Autodesk Fusion 360 part; units mm, degrees
sketch "Sketch1" plane through (0, 0, 0) normal (0, 0, 1) x (1, 0, 0)
  line L0 (0.0319, -0.0588) -> (7.7319, -0.0588)
  line L1 (0.0319, 17.6912) -> (0.0319, -0.0588)
  line L2 (0.0319, 17.6912) -> (5.3319, 17.6912)
  line L3 (0.0319, 8.7412) -> (4.5319, 8.7412)
  line L4 (4.5319, 10.9412) -> (0.0319, 10.9412)
  spline S0 degree 5 poles (5.3319, 17.6912) (5.3878, 17.5532) (5.4935, 17.2775) (5.633, 16.8647) (5.7805, 16.3159) (5.8962, 15.6328) (5.9374, 14.9527) (5.8981, 14.2761) (5.7753, 13.6028) (5.5729, 12.9329) (5.297, 12.2661) (5.0223, 11.7348) (4.7879, 11.3376) (4.6193, 11.0732) (4.5319, 10.9412) knots 0 0 0 0 0 0 0.1 0.2 0.3 0.4 0.5 0.6 0.7 0.8 0.9 1 1 1 1 1 1
  line L5 (0.0319, 10.9412) -> (4.5319, 10.9412)
  arc A0 (7.7319, -0.0588) -> (4.5319, 8.7412) centre (-3.0926, 0.9869) ccw
  line L6 (4.5319, 8.7412) -> (4.5319, 10.9412)
  line L7 (0.0319, 10.9412) -> (0.0319, 8.7412)
  line L8 (0.0319, 10.9412) -> (0.0319, 8.7412)
  line L9 (0.0319, 14.3162) -> (5.8819, 14.3162)
  line L10 (0.0319, 17.6912) -> (0.0319, 10.9412)
  line L11 (7.7319, -0.0588) -> (7.9819, -0.0588)
  line L12 (4.5319, 8.7412) -> (4.7819, 8.7412)
  line L13 (4.5319, 10.9412) -> (4.7819, 10.9412)
  line L14 (5.8819, 14.3162) -> (6.1319, 14.3162)
  line L15 (5.3319, 17.6912) -> (5.5819, 17.6912)
  spline S1 degree 5 poles (5.5819, 17.6912) (5.6378, 17.5532) (5.7435, 17.2775) (5.883, 16.8647) (6.0305, 16.3159) (6.1462, 15.6328) (6.1874, 14.9527) (6.1481, 14.2761) (6.0253, 13.6028) (5.8229, 12.9329) (5.547, 12.2661) (5.2723, 11.7348) (5.0379, 11.3376) (4.8693, 11.0732) (4.7819, 10.9412) knots 0 0 0 0 0 0 0.1 0.2 0.3 0.4 0.5 0.6 0.7 0.8 0.9 1 1 1 1 1 1
  line L16 (4.7819, 10.9412) -> (4.7819, 8.7412)
  arc A1 (7.9819, -0.0588) -> (4.7819, 8.7412) centre (-2.9749, 0.9388) ccw
  line L17 (5.5819, 17.6912) -> (9, 17.6912)
  line L18 (9, 17.6912) -> (12, 17.6912)
  line L19 (12, 17.6912) -> (12, 0)
  line L20 (12, 0) -> (7.9819, -0.0588)
  dimension "d1" = 5.3
  dimension "d2" = 6.75
  dimension "d3" = 4.5
  dimension "d4" = 5.85
  dimension "d5" = 7.7
  dimension "d6" = 11
  dimension "d7" = 2.2
  dimension "d8" = 0.25
  dimension "d9" = 0.25
  dimension "d10" = 0.25
  dimension "d11" = 0.25
  dimension "d12" = 0.25
revolve "Revolve1" add sketch "Sketch1" angle 360 about axis through (0.0319, 17.6912, 0) along (0, -1, 0) contours S1 L16 A1 L17 L18 L19 L20
sketch "Sketch2" plane through (0, 0, 0) normal (1, 0, 0) x (0, 1, 0)
  line L0 (25.8736, 15.4962) -> (-4, 15.4962)
  line L1 (-4, 15.4962) -> (-4, 0)
  line L2 (-4, 0) -> (25.8736, 0)
  line L3 (25.8736, 0) -> (25.8736, 15.4962)
extrude "Extrude1" cut sketch "Sketch2" along normal mid plane 100
sketch "Sketch3" plane through (0, 17.6912, 0) normal (0, 1, 0) x (-1, 0, 0)
  line L0 (11.9363, 0) -> (5.5181, 0)
  arc A0 (-5.5819, 0) -> (5.5181, 0) centre (-0.0319, 0) ccw
  line L1 (-5.5819, 0) -> (-12, 0)
  arc A1 (-12, 0) -> (11.9363, 0) centre (-0.0319, 0) ccw
  line L2 (-12, 0) -> (12.6512, 0)
  line L3 (12.6512, 0) -> (12.6512, -13)
  line L4 (12.6512, -13) -> (-12, -13)
  line L5 (-12, -13) -> (-12, 0)
  circle A2 centre (-0.0319, 0) radius 5.55
  dimension "d16" = 13
extrude "Extrude2" add sketch "Sketch3" against normal blind 17.691 contours A1 L2 L3 L4 L5
sketch "Sketch4" plane through (12, 0, 0) normal (1, 0, 0) x (0, 1, 0)
  line L0 (17.6912, -13) -> (17.6912, 0)
  line L1 (17.6912, 0) -> (0.0002, 0)
  line L2 (0.0002, 0) -> (0.0002, -13)
  line L3 (0.0002, -13) -> (17.6912, -13)
  line L4 (0.0002, 0) -> (-2.6841, 0)
  line L5 (-2.6841, 0) -> (-2.6841, -13)
  line L6 (-2.6841, -13) -> (0.0002, -13)
  line L7 (0.0002, -13) -> (0.0002, 0)
extrude "Extrude3" cut sketch "Sketch4" along normal mid plane 200 contours L2 L4 L5 L6 L7
sketch "Sketch5" plane through (0, 0, 0) normal (0, 0, 1) x (-1, 0, 0)
  line L0 (12.6512, -0.0002) -> (7.9234, -0.0002)
  arc A0 (4.7181, -8.7412) -> (7.9234, -0.0002) centre (-3.0386, -0.9388) ccw
  line L1 (4.7181, -8.7412) -> (4.7181, -10.9412)
  spline S0 degree 3 poles (5.5181, -17.6912) (5.7729, -17.0634) (5.9669, -16.3949) (6.1465, -14.9938) (6.1035, -14.3577) (5.7383, -12.6271) (5.1773, -11.6346) (4.7181, -10.9412) knots -0.494391 -0.494391 -0.494391 -0.494391 -0.376445 -0.376445 -0.249507 -0.249507 0 0 0 0
  line L2 (5.5181, -17.6912) -> (12.6512, -17.6912)
  line L3 (12.6512, -17.6912) -> (12.6512, -0.0002)
  line L4 (12.6512, -17.6912) -> (12.6512, -0.0002)
  line L5 (12.6512, -8.8457) -> (-12, -8.8457)
  line L6 (-12, -8.8457) -> (-12, -17.6912)
  circle A1 centre (8.6512, -8.8457) radius 1.5
  circle A2 centre (-8, -8.8457) radius 1.5
  dimension "d21" = 3
  dimension "d22" = 3
  dimension "d23" = 4
  dimension "d24" = 4
extrude "Extrude4" cut sketch "Sketch5" against normal through all contours L5 A2 | L5 A2 | L5 A1 | L5 A1
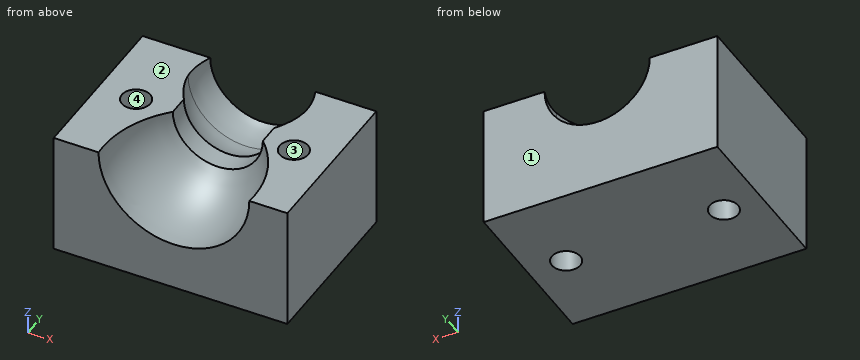
Source: CAD feature listing. Evaluate the final solid. Frame: model axes, mm. Face numbers are marked on the shaded views. Give positions to 0.01 mm unless a question says otherwise; leave off trailing zeros. Write each loop counter-clockwise with the first axis right and the second up, starting at its lowest first coordinate (ties: lowest second). Pieces come first, ordered by that corner, then holes. Notation, with made-up numbers: M 72.5,36 L 108.5,36 A9 ccw 108.5,53 Z; hole C -17,-11 d6. An arc over 180 degrees is marked long. Return JSON: item names as keys, results as strings. Group by question number.
1) Cut plane C-C, the plane z = -2.5. Give the number of separate pieces and of enclosed holes in the cut face, then the cut area to 3 significant figures.
2) First-contact query: pin 1 Ø2.5 at (x, y) = (-8.65, 8.85) entering from -Z (3 decimals); pin 2 Ø1.5 at (x, y) = (2, 2) entering from +Z. Flat tips, straight axial feed; report the tip coordinate or a pass-through.
3) Ray query, L1, parallel to X at y = 8.75, z = -9; L2, parallel to Y at x = 8, z = -3.75; L3, parallel to X at y = 7.5, z = -4.5. Return the intervals inside material, ascending.
4) Cut plane A-A, the plane x = 9. Output: boundary loops of the cut face in (y, z), then the cut area to 3 significant figures.
5) Cut plane B-B, the plane z = -11.75. Output: boundary loops of the cut face in (x, y), then the cut area to 3 significant figures.
6) Draft query along Y for the marked faces 1, 2, 3 and 4. Return one class per face: released by +Y, released by -Y, zero draft, split by the parting line, or undercut.
Data:
{
 "1": {"separate pieces": "2", "enclosed holes": "2", "area": "218 mm²"},
 "2": {"pin 1": "passes through", "pin 2": "stops at z = -7.45"},
 "3": {"L1": "x = -12.65 to -10.15, -7.15 to 6.5, 9.5 to 12", "L2": "y = 0 to 7.35, 10.35 to 17.69", "L3": "x = -12.65 to -9.31, -7.99 to -3.67, 3.73 to 7.34, 8.66 to 12"},
 "4": {"outline": "M 0,-13 L 7.73,-13 L 7.73,0 L 0,0 Z; M 9.96,-13 L 17.69,-13 L 17.69,0 L 9.96,0 Z", "area": "201 mm²"},
 "5": {"outline": "M -12.65,0 L 12,0 L 12,17.69 L -12.65,17.69 Z; hole C -8.65,8.85 d3; hole C 8,8.85 d3", "area": "422 mm²"},
 "6": {"face 1": "released by +Y", "face 2": "zero draft", "face 3": "undercut", "face 4": "undercut"}
}
